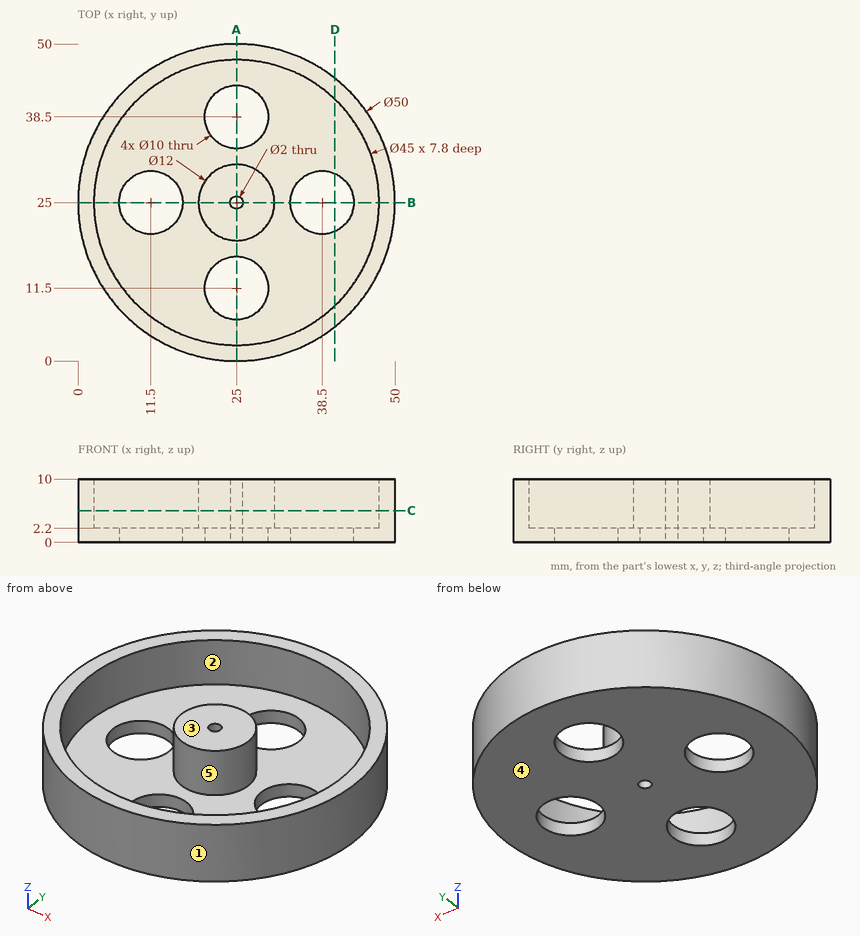
Job drawing, mm, ordinate dimensions from the low corner. One solid piece. A direction names the side the tool comes from. Coordinates: 2 decimals unless noted, no trailing zeros. Write each loop counter-clockwise with the first axis right and the second up, starting at its lowest first coordinate (ties: lowest second). Pieces come first, ordered by that corner, then holes. Notation, with made-up numbers: (79.25, -32.5) - (90.25, -32.5) arc R19 cw to (90.25, -0.5) - close; hole circle Ø1 at (31, -34). An arc over 180 degrees is marked (long way). Use a Markdown table: item, result. Add a question column.
Item 1: Mould opens along X. For the marked faces 1, 2 and 3 say: pulls with the +X half, pulls with the -X half, needs draft (parallel to the pull), parting line crosses it, or undercut.
Item 2: Band-saw the part on D-D, the plane x = 40.5. Give the cut face in (y, z), and give its area (3 significant figures).
Item 3: Band-saw the part on C-C, the plane z = 5. Give the cut face in (x, y), and give its area (3 significant figures).
Item 4: Drill centre lines: L1, parallel to Y at x = 25, z = 1.1; L2, parallel to X at y = 22, z = 1.5; L3, parallel to X at y = 23, z = 1. Where is each one in solid material? Low to high. Write a range as from..to.
Item 5: 3-axis set-ups, long thin cutter, end or side, ignore diameter. For the marked faces 4 and 5: which of +Z, -Z, +X, -X, +Y, -Y reach the whole face in a straight line?
Item 6: Flat gauge pins, fed straight in: pin 1 (1 mm diameter, centred on x = 19, z = 7, fed in from +Y); pin 2 (16 mm diameter, centred on x = 38.5, y = 25, fed in from +Z); pin 3 (4 mm diameter, centred on y = 34, z = 8.5, fed in from -X); pin 4 (8 mm diameter, centred on x = 25, y = 38.5, fed in from -Z). Where does each tip first touch, or does it go through?
Item 7: Band-saw the part on A-A, the plane x = 25. Give the cut face in (y, z).
Numbers:
| question | item | result |
|---|---|---|
| 1 | face 1 | parting line crosses it |
| 1 | face 2 | undercut |
| 1 | face 3 | needs draft |
| 2 | outline | (5.38, 0) - (20.42, 0) - (20.42, 2.2) - (8.69, 2.2) - (8.69, 10) - (5.38, 10) - close; (29.58, 0) - (44.62, 0) - (44.62, 10) - (41.31, 10) - (41.31, 2.2) - (29.58, 2.2) - close |
| 2 | area | 118 mm2 |
| 3 | outline | circle Ø50 at (25, 25); circle Ø12 at (25, 25); hole circle Ø45 at (25, 25); hole circle Ø2 at (25, 25) |
| 3 | area | 483 mm2 |
| 4 | L1 | 0..6.5, 16.5..24, 26..33.5, 43.5..50 |
| 4 | L2 | 0.18..7.5, 15.5..34.5, 42.5..49.82 |
| 4 | L3 | 0.08..6.92, 16.08..33.92, 43.08..49.92 |
| 5 | face 4 | -Z, +X, -X, +Y, -Y |
| 5 | face 5 | +Z |
| 6 | pin 1 | y = 49.39 |
| 6 | pin 2 | z = 10 |
| 6 | pin 3 | x = 1 |
| 6 | pin 4 | through |
| 7 | outline | (0, 0) - (6.5, 0) - (6.5, 2.2) - (2.5, 2.2) - (2.5, 10) - (0, 10) - close; (16.5, 0) - (24, 0) - (24, 10) - (19, 10) - (19, 2.2) - (16.5, 2.2) - close; (26, 0) - (33.5, 0) - (33.5, 2.2) - (31, 2.2) - (31, 10) - (26, 10) - close; (43.5, 0) - (50, 0) - (50, 10) - (47.5, 10) - (47.5, 2.2) - (43.5, 2.2) - close |
